Geometry check sheet. Reference: drawing and pictorial views, mm from the part's lowest x, y, z. Round coordinates to 2 decimals unless told otherwise and drop trailing zeros. Write each loop counter-clockwise with the first axis right and the second up, starting at its lowest first coordinate (ties: lowest second). Pieces come first, ordered by that corner, then holes. Notation, with made-up numbers: (88, 29.25) -> (145, 29.25) arc R6 cw to (145, 40.25) -> close; hole circle Ø3 at (88, 32). An arc over 180 degrees is marked (long way). Write item = value, one per line.
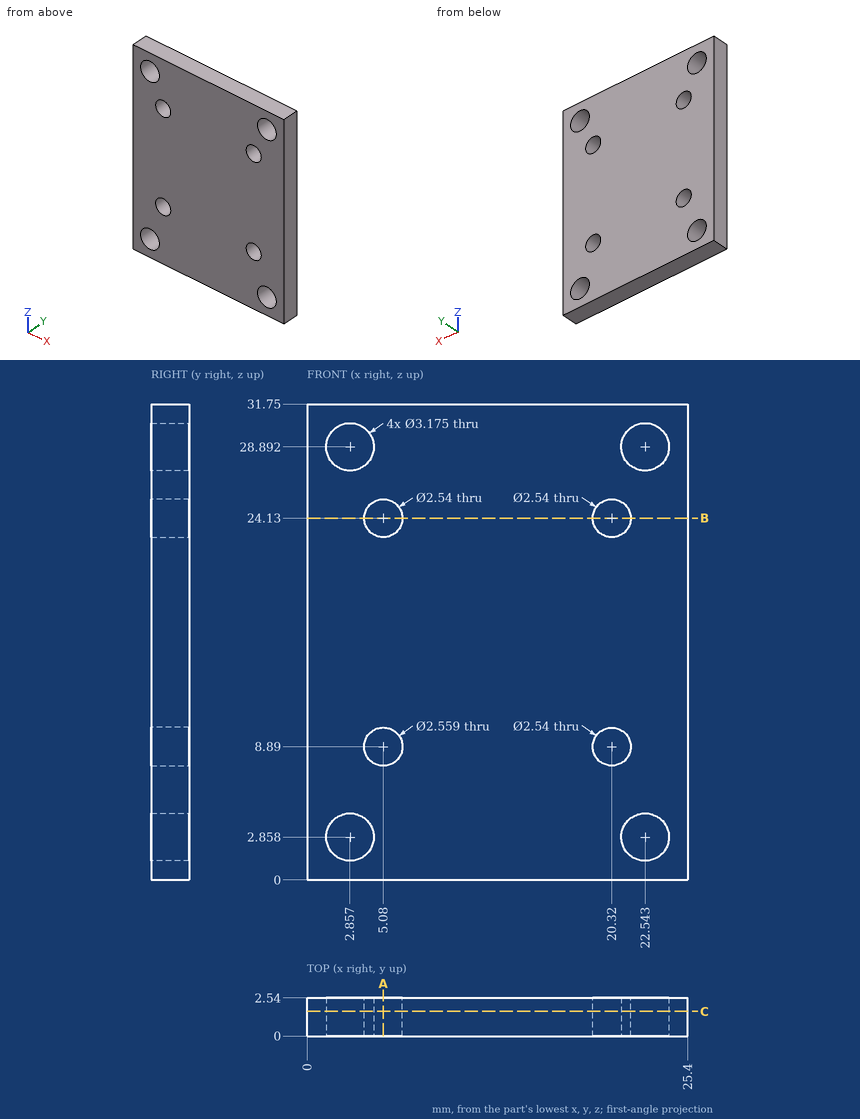
(1) Sectioned sample at C-C on y = 1.65. Count the separate pieces of the cut face and the enclosed holes in it.
Worked answers:
separate_pieces = 1
enclosed_holes = 8
(2) Material ranges on L1, parallel to X at y = 1.85, z = 29; L2, parallel to X at y = 1.2, z = 8.89; L3, parallel to Z at x = 22.25, y = 2.25, recorded low to high. Write a range as [from, to].
Worked answers:
L1 = [0, 1.27], [4.44, 20.96], [24.13, 25.4]
L2 = [0, 3.8], [6.36, 19.05], [21.59, 25.4]
L3 = [0, 1.3], [4.42, 27.33], [30.45, 31.75]
(3) Sectioned sample at A-A on x = 5.08. Enter the section's corners in (y, z).
Worked answers:
outline = (0, 0) -> (2.54, 0) -> (2.54, 7.61) -> (0, 7.61) -> close; (0, 10.17) -> (2.54, 10.17) -> (2.54, 22.86) -> (0, 22.86) -> close; (0, 25.4) -> (2.54, 25.4) -> (2.54, 31.75) -> (0, 31.75) -> close
(4) Go/stop test with a flat-tipped pin: P1, Ø1.9, axis at x = 22.54, z = 2.86, coming from the +Y side. Record where the tip stops, or that it passes through.
Worked answers:
P1 = through
(5) Sectioned sample at B-B on z = 24.13. Enter the section's corners in (x, y).
Worked answers:
outline = (0, 0) -> (3.81, 0) -> (3.81, 2.54) -> (0, 2.54) -> close; (6.35, 0) -> (19.05, 0) -> (19.05, 2.54) -> (6.35, 2.54) -> close; (21.59, 0) -> (25.4, 0) -> (25.4, 2.54) -> (21.59, 2.54) -> close
